```python
from build123d import *

# Parameters (mm, degrees)
SKETCH1_W           = 30
SKETCH1_H           = 17
BOSS_EXTRUDE1_DEPTH = 4
SKETCH5_W           = 30
SKETCH5_H           = 4
BOSS_EXTRUDE2_DEPTH = 16
CUT_EXTRUDE3_DEPTH  = 10
CUT_EXTRUDE5_DEPTH  = 10


with BuildPart() as part:
    # Sketch1 → Boss-Extrude1 (new body)
    with BuildSketch(Plane(origin=(0, 0, 0), x_dir=(1, 0, 0), z_dir=(0, 1, 0))):
        with Locations((-29.259259259, 2.888888889)):
            Rectangle(SKETCH1_W, SKETCH1_H)
    extrude(amount=BOSS_EXTRUDE1_DEPTH)

    # Sketch5 → Boss-Extrude2 (add)
    with BuildSketch(Plane(origin=(0, 4, 0), x_dir=(1, 0, 0), z_dir=(0, 1, 0))):
        with Locations((-29.259259259, -3.611111111)):
            Rectangle(SKETCH5_W, SKETCH5_H)
    extrude(amount=BOSS_EXTRUDE2_DEPTH)

    # Sketch7 → Cut-Extrude3 (cut)
    with BuildSketch(Plane(origin=(0, 4, 0), x_dir=(1, 0, 0), z_dir=(0, 1, 0))):
        with BuildLine():
            Line((-18.259259259, 5.384968307), (-40.259259259, 5.384968307))
            ThreePointArc((-40.259259259, 5.384968307), (-42.359259259, 7.484968307), (-40.259259259, 9.584968307))
            Line((-40.259259259, 9.584968307), (-18.259259259, 9.584968307))
            ThreePointArc((-18.259259259, 9.584968307), (-16.159259259, 7.484968307), (-18.259259259, 5.384968307))
        make_face()
    extrude(amount=-CUT_EXTRUDE3_DEPTH, mode=Mode.SUBTRACT)

    # Sketch8 → Cut-Extrude5 (cut)
    with BuildSketch(Plane(origin=(0, 0, 1.611111111), x_dir=(-1, 0, 0), z_dir=(0, 0, -1))):
        with BuildLine():
            Line((24.259259259, 11.997218425), (34.259259259, 11.997218425))
            ThreePointArc((34.259259259, 11.997218425), (36.359259259, 9.897218425), (34.259259259, 7.797218425))
            Line((34.259259259, 7.797218425), (24.259259259, 7.797218425))
            ThreePointArc((24.259259259, 7.797218425), (22.159259259, 9.897218425), (24.259259259, 11.997218425))
        make_face()
    extrude(amount=-CUT_EXTRUDE5_DEPTH, mode=Mode.SUBTRACT)


solid = part.part
```
CAD build for the part. Positions are in the model's coordinates, mm. A direction names the side the tool comes from. Round coordinates to 2 decimals unless told otherwise and drop trailing zeros. Loops run counter-clockwise (first coordinate to the right, second up) from the corner with the lowest first, then second, coordinate; pieces in that order, holes last. Notation, with made-up numbers: M 23,-23 L 35,-23 A11 ccw 35,-4 Z; hole C 66.25,-20 d11. An arc over 180 degrees is marked long. Return JSON: item names as keys, results as strings. Group by question number.
(1) Tool access for faces 5 (the flat face through (-29, 2, -5.385)), 6 (the flat face through (-29, 20, 4)), 7 (the flat face through (-29, 11.997, 4)), 8 (the flat face through (-29, 4, -4)), 9 (the flat face through (-29, 0, -1)): list every direction of +Z, -Z, +X, -X, +Y, -Y with a clear straight run to the whole face (end or side of a thin tool).
(2) Saw through at D-D, the plane x = -25. List the corners of the cut face in (y, z), and give its area (3 significant figures).
(3) Wall check: probe 1 along Z at (x, y) = (-39.5, 2.5); probe 2 along Z at (x, y) = (-22, 15.25); probe 3 along Z at (x, y) = (-41, 1.75). Give the ranges that are in metal, low to high. Write a range as [from, to].
(4) Drop flat-ended pins along their axis: P1, Ø5, axis at x = -29.5, y = 12, coming from the -Z side; P2, Ø10, axis at x = -39, z = -7, coming from the +Y side. Give the stop position or say it passes through.
(5) Mould opens along X. For faces 1 (the cylindrical face through (-36.36, 9.94, 3.58)), 2 (the flat face through (-14.259, 5, 3)), 3 (the flat face through (-44.259, 5, 3)), 4 (the flat face through (-29, 14, 1.611)) say: +X half, -X half, draft (parallel to the pull), parting line (faces both ways), or undercut.
(6) Saw through at C-C, the plane y = 2.25. List the corners of the cut face in (x, z), and give its area (3 significant figures).
(7) Saw through at B-B, the plane z = -6.25. List the corners of the cut face in (x, y), and give its area (3 significant figures).
(8) Saw through at A-A, the plane x = -20. List the corners of the cut face in (y, z).
Answer list:
{
 "1": {"face 5": "+Y, -Y", "face 6": "+Z, -Z, +X, -X, +Y", "face 7": "+Z, -Z", "face 8": "-Z, +X, -X, +Y", "face 9": "+Z, -Z, +X, -X, -Y"},
 "2": {"outline": "M 0,-11.39 L 4,-11.39 L 4,-9.58 L 0,-9.58 Z; M 0,-5.38 L 4,-5.38 L 4,1.61 L 7.8,1.61 L 7.8,5.61 L 0,5.61 Z; M 12,1.61 L 20,1.61 L 20,5.61 L 12,5.61 Z", "area": "98.4 mm2"},
 "3": {"probe 1": "[-11.39, -9.58], [-5.38, 5.61]", "probe 2": "[1.61, 5.61]", "probe 3": "[-11.39, -9.45], [-5.52, 5.61]"},
 "4": {"P1": "z = 1.61", "P2": "y = 4"},
 "5": {"face 1": "undercut", "face 2": "+X half", "face 3": "-X half", "face 4": "draft"},
 "6": {"outline": "M -44.26,-11.39 L -14.26,-11.39 L -14.26,5.61 L -44.26,5.61 Z; hole M -40.26,-9.58 L -18.26,-9.58 A2.1 ccw -18.26,-5.38 L -40.26,-5.38 A2.1 ccw Z", "area": "404 mm2"},
 "7": {"outline": "M -44.26,0 L -41.96,0 L -41.96,4 L -44.26,4 Z; M -16.56,0 L -14.26,0 L -14.26,4 L -16.56,4 Z", "area": "18.4 mm2"},
 "8": {"outline": "M 0,-11.39 L 4,-11.39 L 4,-9.58 L 0,-9.58 Z; M 0,-5.38 L 4,-5.38 L 4,1.61 L 20,1.61 L 20,5.61 L 0,5.61 Z"}
}
